Geometry: final body of the model. Coordinates: model frame, mm. A direction names the side the tool comes from. Give positions to 0.01 mm unless a question says otherwise; leave off trailing zeros. Order: outer loops, then holes, each group sorted by start corner. A loop starts at its lowest first (then second) coordinate and runs counter-clockwise, first axis right, second up. Notation, with made-up numbers: (-36, -19.75) -> (21, -19.75) arc R17 ccw to (21, -2.75) -> close; hole circle Ø1 at (-11, 16). An arc over 180 degrees is marked (long way). Answer in a Markdown table with one row per item. Add a question column.
Q1. Pull-direction query (X, two-part tool) for faces 1 (the face through (-35, 70.104, 0)), 2 (the face through (-7.3, 72.37, -0.09)), 3 (the face through (-35, 73.279, 0)); classes: +X half, -X half, draft (parallel to the pull), parting line (faces both ways), or undercut.
Q2. Line query: line 1 along X through (y, z) = (22, 0.25) (3 decimals); line 2 along Z through (x, y) = (0, 1) (3 decimals); line 3 along X through (y, z) = (0.9, 0) (3 decimals). Output: solid intervals per line, ascending. Write a range as from..to.
Q3. Contact query for flat-ended pins moving along their axis: P1, Ø5, axis at x = -69.45, z = 0, coming from the +Y side; P2, Ø3, axis at y = 11.5, z = 0, coming from the +X side; P3, Ø1.5, axis at x = -63.5, z = 0.5, coming from the +Y side; P4, Ø4, axis at y = 42, z = 1.5, coming from the -X side. Output: stop coordinate, or through.
Q4. Cut plane D-D on x = -15.5. Return the cut outline in (y, z), and give its area (3 significant figures).
Q5. Cut plane B-B on z = 0. Count the separate pieces of the cut face and the enclosed holes in it, and give its area (3 significant figures).
Q6. Set-up query: faces 4 (the face through (-59.925, 35, 0)), 5 (the face through (-73, 3.175, 0)), 6 (the face through (-75.8, 2, 0)), 7 (the face through (-6.35, 37, 0)). Return all of +Z, -Z, +X, -X, +Y, -Y with unobstructed straight access to the full face (end or side cutting, diameter ignored); none if empty.
Q7. Cut plane C-C on y = 13. Return the cut outline in (x, z) (3 decimals), and give its area (3 significant figures).
Q8. Cut plane A-A on x = -69.45. Return the cut outline in (y, z) (3 decimals), and give its area (3 significant figures).
from build123d import *

# Parameters (mm, degrees)
SKETCH1_W             = 15.875
SKETCH1_H             = 12.7
SKETCH1_R             = 3.175
BOSS_EXTRUDE1_DEPTH   = 3.175
BOSS_EXTRUDE1_2_DEPTH = 3.175
SKETCH2_W             = 3.175
SKETCH2_H             = 12.7
BOSS_EXTRUDE2_DEPTH   = 70.104
SKETCH3_W             = 3.175
SKETCH3_H             = 12.7
SKETCH3_W_2           = 53.575
BOSS_EXTRUDE3_DEPTH   = 3.175
FILLET5_R             = 3.175
FILLET6_R             = 1.5875


with BuildPart() as part:
    # Sketch1 → Boss-Extrude1 (new body)
    with BuildSketch(Plane(origin=(0, 0, 0), x_dir=(1, 0, 0), z_dir=(0, 1, 0))):
        with Locations((-1.5875, 0)):
            Rectangle(SKETCH1_W, SKETCH1_H)
        Circle(SKETCH1_R, mode=Mode.SUBTRACT)
    extrude(amount=BOSS_EXTRUDE1_DEPTH)



with BuildPart() as body_2:
    # Sketch1 → Boss-Extrude1 2 (new body)
    with BuildSketch(Plane(origin=(0, 0, 0), x_dir=(1, 0, 0), z_dir=(0, 1, 0))):
        with Locations((-67.8625, 0)):
            Rectangle(SKETCH1_W, SKETCH1_H)
        with Locations((-69.45, 0)):
            Circle(SKETCH1_R, mode=Mode.SUBTRACT)
    extrude(amount=BOSS_EXTRUDE1_2_DEPTH)


with BuildPart() as part_1:
    add(part.part)

    add(body_2.part)  # Boss-Extrude2 merges body 2
    # Sketch2 → Boss-Extrude2 (add)
    with BuildSketch(Plane(origin=(0, 3.175, 0), x_dir=(1, 0, 0), z_dir=(0, 1, 0))):
        with Locations((-61.5125, 0)):
            Rectangle(SKETCH2_W, SKETCH2_H)
        with Locations((-7.9375, 0)):
            Rectangle(SKETCH2_W, SKETCH2_H)
    extrude(amount=BOSS_EXTRUDE2_DEPTH)

    # Sketch3 → Boss-Extrude3 (add)
    with BuildSketch(Plane(origin=(0, 73.279, 0), x_dir=(1, 0, 0), z_dir=(0, 1, 0))):
        with Locations((-61.5125, 0)):
            Rectangle(SKETCH3_W, SKETCH3_H)
        with Locations((-33.1375, 0)):
            Rectangle(SKETCH3_W_2, SKETCH3_H)
    extrude(amount=-BOSS_EXTRUDE3_DEPTH)

    # Fillet5
    fillet5_edges = [part_1.edges().sort_by_distance(p)[0] for p in [
        (-63.1, 73.279, 0),
        (-6.35, 73.279, 0),
        (-9.525, 0, 0),
        (-59.925, 0, 0),
    ]]
    fillet(fillet5_edges, radius=FILLET5_R)

    # Fillet6
    fillet6_edges = [part_1.edges().sort_by_distance(p)[0] for p in [
        (-63.1, 3.175, 0),
        (-59.925, 70.104, 0),
        (-9.525, 70.104, 0),
        (-6.35, 3.175, 0),
    ]]
    fillet(fillet6_edges, radius=FILLET6_R)


solid = part_1.part
Completed:
| question | item | result |
|---|---|---|
| 1 | face 1 | undercut |
| 1 | face 2 | +X half |
| 1 | face 3 | draft |
| 2 | line 1 | x = -63.1..-59.925, -9.525..-6.35 |
| 2 | line 2 | z = -6.35..-3.175, 3.175..6.35 |
| 2 | line 3 | x = -75.8..-72.625, -66.275..-60.885, -8.565..-3.175, 3.175..6.35 |
| 3 | P1 | passes through |
| 3 | P2 | stops at x = -6.35 |
| 3 | P3 | stops at y = 71.55 |
| 3 | P4 | stops at x = -63.1 |
| 4 | outline | (70.1, -6.35) -> (73.28, -6.35) -> (73.28, 6.35) -> (70.1, 6.35) -> close |
| 4 | area | 40.3 mm² |
| 5 | separate pieces | 3 |
| 5 | enclosed holes | 0 |
| 5 | area | 659 mm² |
| 6 | face 4 | +Z, -Z, -Y |
| 6 | face 5 | +Z, -Z, -X, +Y |
| 6 | face 6 | +Z, -Z, -X, +Y, -Y |
| 6 | face 7 | +Z, -Z, +X, +Y |
| 7 | outline | (-63.1, -6.35) -> (-59.925, -6.35) -> (-59.925, 6.35) -> (-63.1, 6.35) -> close; (-9.525, -6.35) -> (-6.35, -6.35) -> (-6.35, 6.35) -> (-9.525, 6.35) -> close |
| 7 | area | 80.6 mm² |
| 8 | outline | (0, -6.35) -> (3.175, -6.35) -> (3.175, -3.175) -> (0, -3.175) -> close; (0, 3.175) -> (3.175, 3.175) -> (3.175, 6.35) -> (0, 6.35) -> close |
| 8 | area | 20.2 mm² |
